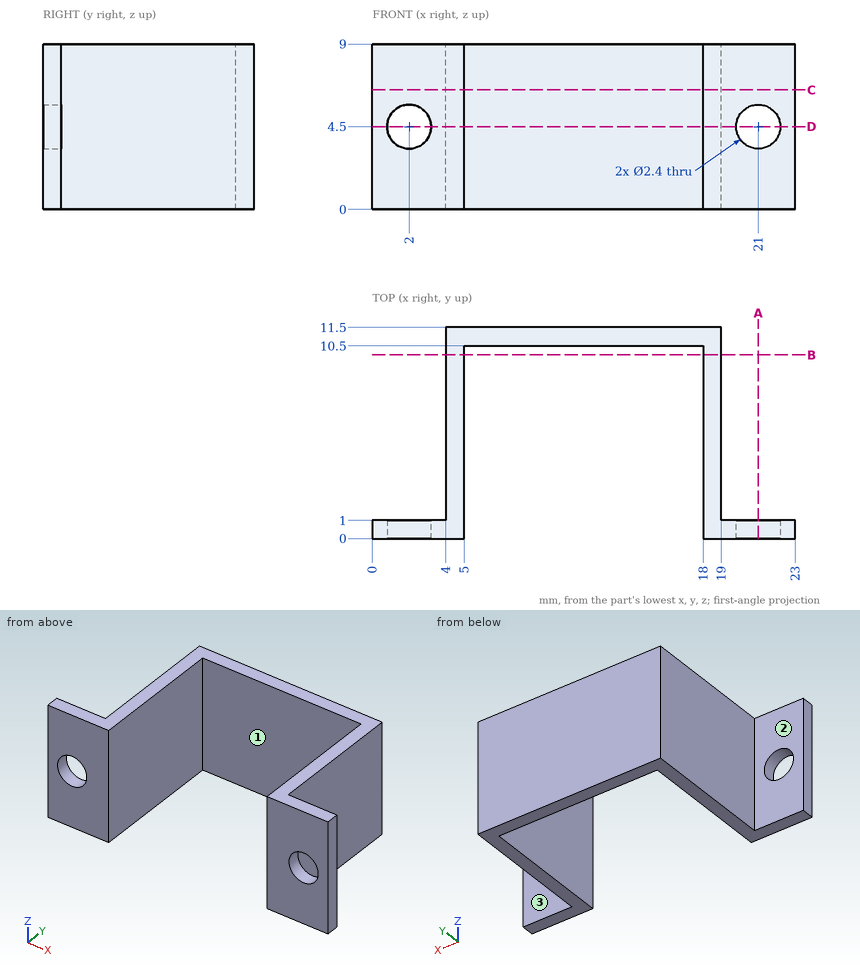
Check sheet for the drawn part. Datum: minimum x, y, z corner. Units: mm. A direction names the side the tool comes from. Coordinates: 2 decimals unless noted, no trailing zeros. Order: outer loops, then holes, each group sorted by start corner. A loop starts at its lowest first (then second) coordinate and runs counter-clockwise, first axis right, second up. Notation, with made-up numbers: M 53,44 L 85,44 A8 cw 85,52 Z; hole C -23,56.25 d9. An arc over 180 degrees is marked long. One line per question, with ' | ' between items. Start each with the question number.
Item 1: Set-up check for the marked faces 1, 2 and 3: record each of +Z, -Z, +X, -X, +Y, -Y from which the full face is reachable in a straight line by a thin tool's end or side.
Item 2: Cross-section at A-A on x = 21. Enter the section's corners in (y, z), then the cut area to 3 significant figures.
Item 3: Cross-section at C-C on z = 6.5. Enter the section's corners in (x, y).
Item 4: Material ranges on L1, parallel to X at y = 0.35, z = 4.5; L2, parallel to X at y = 5.5, z = 7.5; L3, parallel to Z at x = 2, y = 0.85, recorded low to high. Write a range as [from, to].
Item 5: Cross-section at D-D on z = 4.5. Enter the section's corners in (x, y).
Item 6: Cross-section at B-B on y = 10. Enter the section's corners in (x, z).
Item 7: Gauge pin test, flat ends, axial feed: pin 1 (2.5 mm diameter, centred on x = 10.5, z = 3.5, fed in from -Y); pin 2 (2.5 mm diameter, centred on y = 4.5, z = 3, fed in from -X); pin 3 (3 mm diameter, centred on x = 21, z = 4.5, fed in from -Y); pin 4 (3 mm diameter, centred on x = 2, z = 5.5, fed in from +Y). Record the tip position at first contact, or that the pin passes through.
Findings:
1) face 1: +Z, -Z, -Y | face 2: +Z, -Z, -X, +Y | face 3: +Z, -Z, +X, +Y
2) outline: M 0,0 L 1,0 L 1,3.3 L 0,3.3 Z; M 0,5.7 L 1,5.7 L 1,9 L 0,9 Z | area: 6.60 mm²
3) outline: M 0,0 L 5,0 L 5,10.5 L 18,10.5 L 18,0 L 23,0 L 23,1 L 19,1 L 19,11.5 L 4,11.5 L 4,1 L 0,1 Z
4) L1: x = [0, 0.8], [3.2, 5], [18, 19.8], [22.2, 23] | L2: x = [4, 5], [18, 19] | L3: z = [0, 3.3], [5.7, 9]
5) outline: M 0,0 L 0.8,0 L 0.8,1 L 0,1 Z; M 3.2,0 L 5,0 L 5,10.5 L 18,10.5 L 18,0 L 19.8,0 L 19.8,1 L 19,1 L 19,11.5 L 4,11.5 L 4,1 L 3.2,1 Z; M 22.2,0 L 23,0 L 23,1 L 22.2,1 Z
6) outline: M 4,0 L 5,0 L 5,9 L 4,9 Z; M 18,0 L 19,0 L 19,9 L 18,9 Z
7) pin 1: stops at y = 10.5 | pin 2: stops at x = 4 | pin 3: stops at y = 0 | pin 4: stops at y = 1
